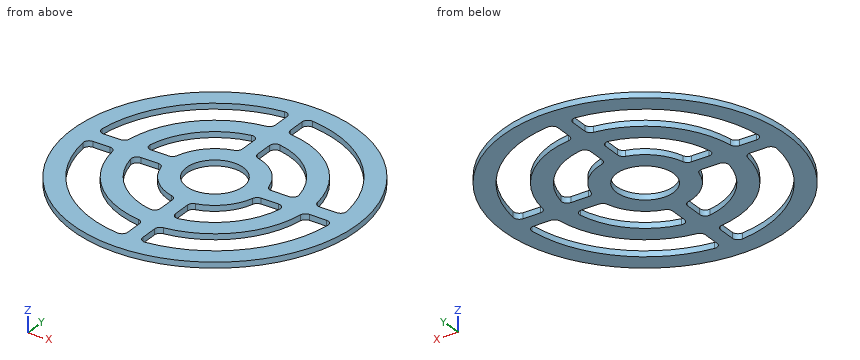
from build123d import *

# Parameters (mm, degrees)
F0_R     = 75
F0_R_2   = 15
F1_DEPTH = 3
F2_R     = 3


with BuildPart() as f1:
    # F0 (on Top) → F1 (new body)
    with BuildSketch(Plane.XY):
        Circle(F0_R)
        with BuildLine():
            ThreePointArc((4, 64.876806), (45.961941, 45.961941), (64.876806, 4))
            ThreePointArc((64.876806, 4), (64.969194, 2.000948), (65, 0))
            ThreePointArc((65, 0), (64.969194, -2.000948), (64.876806, -4))
            ThreePointArc((64.876806, -4), (45.961941, -45.961941), (4, -64.876806))
            ThreePointArc((4, -64.876806), (0, -65), (-4, -64.876806))
            ThreePointArc((-4, -64.876806), (-45.961941, -45.961941), (-64.876806, -4))
            ThreePointArc((-64.876806, -4), (-65, 0), (-64.876806, 4))
            ThreePointArc((-64.876806, 4), (-45.961941, 45.961941), (-4, 64.876806))
            ThreePointArc((-4, 64.876806), (0, 65), (4, 64.876806))
        make_face(mode=Mode.SUBTRACT)
        with BuildLine():
            ThreePointArc((-4, 49.839743), (0, 50), (4, 49.839743))
            Line((4, 49.839743), (4, 64.876806))
            ThreePointArc((4, 64.876806), (0, 65), (-4, 64.876806))
            Line((-4, 64.876806), (-4, 49.839743))
        make_face()
        with BuildLine():
            ThreePointArc((49.839743, -4), (49.95992, -2.001604), (50, 0))
            ThreePointArc((50, 0), (49.95992, 2.001604), (49.839743, 4))
            ThreePointArc((49.839743, 4), (35.355339, 35.355339), (4, 49.839743))
            ThreePointArc((4, 49.839743), (0, 50), (-4, 49.839743))
            ThreePointArc((-4, 49.839743), (-35.355339, 35.355339), (-49.839743, 4))
            ThreePointArc((-49.839743, 4), (-50, 0), (-49.839743, -4))
            ThreePointArc((-49.839743, -4), (-35.355339, -35.355339), (-4, -49.839743))
            ThreePointArc((-4, -49.839743), (0, -50), (4, -49.839743))
            ThreePointArc((4, -49.839743), (35.355339, -35.355339), (49.839743, -4))
        make_face()
        with BuildLine():
            ThreePointArc((39.799497, 4), (39.949843, 2.002511), (40, 0))
            ThreePointArc((40, 0), (39.949843, -2.002511), (39.799497, -4))
            ThreePointArc((39.799497, -4), (28.284271, -28.284271), (4, -39.799497))
            ThreePointArc((4, -39.799497), (0, -40), (-4, -39.799497))
            ThreePointArc((-4, -39.799497), (-28.284271, -28.284271), (-39.799497, -4))
            ThreePointArc((-39.799497, -4), (-40, 0), (-39.799497, 4))
            ThreePointArc((-39.799497, 4), (-28.284271, 28.284271), (-4, 39.799497))
            ThreePointArc((-4, 39.799497), (0, 40), (4, 39.799497))
            ThreePointArc((4, 39.799497), (28.284271, 28.284271), (39.799497, 4))
        make_face(mode=Mode.SUBTRACT)
        with BuildLine():
            Line((4, 24.677925), (4, 39.799497))
            ThreePointArc((4, 39.799497), (0, 40), (-4, 39.799497))
            Line((-4, 39.799497), (-4, 24.677925))
            ThreePointArc((-4, 24.677925), (0, 25), (4, 24.677925))
        make_face()
        with BuildLine():
            ThreePointArc((25, 0), (24.919351, 2.006473), (24.677925, 4))
            ThreePointArc((24.677925, 4), (17.67767, 17.67767), (4, 24.677925))
            ThreePointArc((4, 24.677925), (0, 25), (-4, 24.677925))
            ThreePointArc((-4, 24.677925), (-17.67767, 17.67767), (-24.677925, 4))
            ThreePointArc((-24.677925, 4), (-25, 0), (-24.677925, -4))
            ThreePointArc((-24.677925, -4), (-17.67767, -17.67767), (-4, -24.677925))
            ThreePointArc((-4, -24.677925), (0, -25), (4, -24.677925))
            ThreePointArc((4, -24.677925), (17.67767, -17.67767), (24.677925, -4))
            ThreePointArc((24.677925, -4), (24.919351, -2.006473), (25, 0))
        make_face()
        Circle(F0_R_2, mode=Mode.SUBTRACT)
        with BuildLine():
            Line((-24.677925, 4), (-39.799497, 4))
            ThreePointArc((-39.799497, 4), (-40, 0), (-39.799497, -4))
            Line((-39.799497, -4), (-24.677925, -4))
            ThreePointArc((-24.677925, -4), (-25, 0), (-24.677925, 4))
        make_face()
        with BuildLine():
            ThreePointArc((-49.839743, -4), (-50, 0), (-49.839743, 4))
            Line((-49.839743, 4), (-64.876806, 4))
            ThreePointArc((-64.876806, 4), (-65, 0), (-64.876806, -4))
            Line((-64.876806, -4), (-49.839743, -4))
        make_face()
        with BuildLine():
            ThreePointArc((-4, -39.799497), (0, -40), (4, -39.799497))
            Line((4, -39.799497), (4, -24.677925))
            ThreePointArc((4, -24.677925), (0, -25), (-4, -24.677925))
            Line((-4, -24.677925), (-4, -39.799497))
        make_face()
        with BuildLine():
            Line((4, -64.876806), (4, -49.839743))
            ThreePointArc((4, -49.839743), (0, -50), (-4, -49.839743))
            Line((-4, -49.839743), (-4, -64.876806))
            ThreePointArc((-4, -64.876806), (0, -65), (4, -64.876806))
        make_face()
        with BuildLine():
            ThreePointArc((39.799497, -4), (39.949843, -2.002511), (40, 0))
            ThreePointArc((40, 0), (39.949843, 2.002511), (39.799497, 4))
            Line((39.799497, 4), (24.677925, 4))
            ThreePointArc((24.677925, 4), (24.919351, 2.006473), (25, 0))
            ThreePointArc((25, 0), (24.919351, -2.006473), (24.677925, -4))
            Line((24.677925, -4), (39.799497, -4))
        make_face()
        with BuildLine():
            ThreePointArc((49.839743, 4), (49.95992, 2.001604), (50, 0))
            ThreePointArc((50, 0), (49.95992, -2.001604), (49.839743, -4))
            Line((49.839743, -4), (64.876806, -4))
            ThreePointArc((64.876806, -4), (64.969194, -2.000948), (65, 0))
            ThreePointArc((65, 0), (64.969194, 2.000948), (64.876806, 4))
            Line((64.876806, 4), (49.839743, 4))
        make_face()
    extrude(amount=F1_DEPTH)

    # F2
    f2_edges = [f1.edges().sort_by_distance(p)[0] for p in [
        (-64.876806, 4, 1.5),
        (-39.799497, 4, 1.5),
        (4, 24.677925, 1.5),
        (49.839743, 4, 1.5),
        (24.677925, 4, 1.5),
        (4, -39.799497, 1.5),
        (4, -64.876806, 1.5),
        (4, 49.839743, 1.5),
        (64.876806, -4, 1.5),
        (39.799497, -4, 1.5),
        (-4, 39.799497, 1.5),
        (-4, -24.677925, 1.5),
        (-4, -49.839743, 1.5),
        (-49.839743, -4, 1.5),
        (-4, 64.876806, 1.5),
        (4, 64.876806, 1.5),
        (-64.876806, -4, 1.5),
        (-39.799497, -4, 1.5),
        (24.677925, -4, 1.5),
        (49.839743, -4, 1.5),
        (4, -49.839743, 1.5),
        (-4, -64.876806, 1.5),
        (-4, -39.799497, 1.5),
        (-24.677925, 4, 1.5),
        (39.799497, 4, 1.5),
        (64.876806, 4, 1.5),
        (-4, 24.677925, 1.5),
        (-4, 49.839743, 1.5),
        (-49.839743, 4, 1.5),
        (4, -24.677925, 1.5),
        (4, 39.799497, 1.5),
        (-24.677925, -4, 1.5),
    ]]
    fillet(f2_edges, radius=F2_R)


solid = f1.part
Could you check a few things on this model? Use its own coordinates, in mm. Coordinates: 2 decimals unless noted, no trailing zeros. Order: outer loops, then holes, each group sorted by start corner. A loop starts at its lowest first (then second) coordinate and runs counter-clockwise, first axis right, second up. Notation, with made-up numbers: (57, 20.25) -> (115, 20.25) arc R25 ccw to (115, 39.25) -> close; hole circle Ø2 at (73.25, 25). An arc over 180 degrees is marked (long way). One line per item, written item: value. Start each with the question number.
1) Imagine slicing it at A-A on x = 0. List the corners of the cut face in (y, z) for me, plus the area to 3 significant figures.
2) Imagine slicing it at C-C on y = 33.5. List the corners of the cut face in (x, z) for me, plus the area to 3 significant figures.
3) Imagine slicing it at D-D on x = -33. List the corners of the cut face in (y, z) for me.
4) If I drill on L1, parallel to Y at x = -28, z = 2.8; L2, parallel to Y at x = 36, z = 1.7; L3, parallel to Y at x = -8, z = 1.5, over which ranges is the centre line in solid material (lowest first)? Write a range as [from, to].
5) I'm going to push flat-ended pins straight in: pin 1 (0.9 mm diameter, centred on y = -58, z = 2, fed in from -X); pin 2 (0.9 mm diameter, centred on y = -33, z = 1.5, fed in from +X); pin 3 (0.9 mm diameter, centred on x = -56.5, z = 2, fed in from +Y). Where does each tip first touch, or does it pass through?
Answer list:
1. outline: (-75, 0) -> (-15, 0) -> (-15, 3) -> (-75, 3) -> close; (15, 0) -> (75, 0) -> (75, 3) -> (15, 3) -> close
1. area: 360 mm2
2. outline: (-67.1, 0) -> (-55.7, 0) -> (-55.7, 3) -> (-67.1, 3) -> close; (-37.12, 0) -> (-21.86, 0) -> (-21.86, 3) -> (-37.12, 3) -> close; (-4, 0) -> (4, 0) -> (4, 3) -> (-4, 3) -> close; (21.86, 0) -> (37.12, 0) -> (37.12, 3) -> (21.86, 3) -> close; (55.7, 0) -> (67.1, 0) -> (67.1, 3) -> (55.7, 3) -> close
2. area: 184 mm2
3. outline: (-67.35, 0) -> (-56, 0) -> (-56, 3) -> (-67.35, 3) -> close; (-37.56, 0) -> (-22.61, 0) -> (-22.61, 3) -> (-37.56, 3) -> close; (-4, 0) -> (4, 0) -> (4, 3) -> (-4, 3) -> close; (22.61, 0) -> (37.56, 0) -> (37.56, 3) -> (22.61, 3) -> close; (56, 0) -> (67.35, 0) -> (67.35, 3) -> (56, 3) -> close
4. L1: y = [-69.58, -58.66], [-41.42, -28.57], [-4, 4], [28.57, 41.42], [58.66, 69.58]
4. L2: y = [-65.8, -54.12], [-34.7, -17.44], [-4, 4], [17.44, 34.7], [54.12, 65.8]
4. L3: y = [-74.57, -64.51], [-49.36, -39.19], [-23.69, -12.69], [12.69, 23.69], [39.19, 49.36], [64.51, 74.57]
5. pin 1: stops at x = -48.09
5. pin 2: stops at x = 67.57
5. pin 3: stops at y = 49.83
